Here's how the part is built. I have some questions about the finished solid (model axes, mm). Face numbers are marked on the shaded views. A direction names the side the tool comes from. Round coordinates to 2 decimals unless told otherwise and drop trailing zeros. Order: outer loops, then holes, each group sorted by start corner. A loop starts at its lowest first (then second) coordinate and runs counter-clockwise, first axis right, second up. Notation, with made-up numbers: (-18, 83.5) -> (-4, 83.5) arc R28 cw to (-4, 103.5) -> close; hole circle Ø5 at (-19, 85.5). An arc over 180 degrees is marked (long way). Use a Markdown table: item, result. Add a question column.
(1) Thinking about a two-plate mould opening in X: for the marked faces 4, 5, 6 and 7, which applies, pulls with the +X half, pulls with the -X half, needs draft (parallel to the pull), parting line crosses it, or undercut?
(2) I want a section at A-A, the plane z = 2.7. Please give me the cut outline in (x, y) (3 decimals).
(3) I want a section at B-B, the plane x = 2.75. Please give me the cut outline in (y, z).
(4) If I drill on probe 1 along Y at (x, z) = (5, 4.35) (3 decimals); probe 2 along X at (y, z) = (7.25, 2.9); probe 3 along X at (y, z) = (12.25, 3.3), over which ranges is the centre line in solid material (lowest first)?
(5) I want a section at C-C, the plane y = 11.25. Please give me the cut outline in (x, z), then the cut area to 3 significant figures.
(6) On a 3-axis mill with a long thin cutter (end or side, diameter ignored), from which of +Z, -Z, +X, -X, +Y, -Y can I reach the whole of each face in a straight line? I mean the marked faces 1, 2 and 3. Say none if no direction works.
(7) I want a section at D-D, the plane x = 5. Please give me the cut outline in (y, z) (3 decimals), then the cut area to 3 significant figures.
(8) I'm going to push flat-ended pins straight in: P1, Ø0.9, axis at y = 13.5, z = 4, coming from the -X side; P2, Ø1, axis at y = 4, z = 3, coming from the -X side; P3, Ø1.2, axis at y = 13.5, z = 2.5, coming from the +X side; P4, Ø5, axis at x = 8.5, y = 11.5, coming from the -Z side. Where does each tip first touch, or does it pass through?
from build123d import *

# Parameters (mm, degrees)
SKETCH1_R           = 3.5
BOSS_EXTRUDE1_DEPTH = 6
SKETCH2_W           = 3
SKETCH2_H           = 6
CUT_EXTRUDE1_DEPTH  = 23.414057106
FILLET1_R           = 2
FILLET2_R           = 1


with BuildPart() as part:
    # Sketch1 → Boss-Extrude1 (new body)
    with BuildSketch(Plane.XY):
        with BuildLine():
            Line((0, 3), (0, 0))
            Line((0, 0), (10, 0))
            Line((10, 0), (10, 3))
            ThreePointArc((10, 3), (5, 17.244997998), (0, 3))
        make_face()
        with Locations((5, 9.244997998)):
            Circle(SKETCH1_R, mode=Mode.SUBTRACT)
    extrude(amount=BOSS_EXTRUDE1_DEPTH)

    # Sketch2 → Cut-Extrude1 (cut, through all)
    with BuildSketch(Plane.XY.offset(6)):
        with Locations((5, 15)):
            Rectangle(SKETCH2_W, SKETCH2_H)
    extrude(amount=-CUT_EXTRUDE1_DEPTH, mode=Mode.SUBTRACT)

    # Fillet1
    fillet1_edges = [part.edges().sort_by_distance(p)[0] for p in [
        (3.5, 17.103114821, 3),
        (6.5, 17.103114821, 3),
    ]]
    fillet(fillet1_edges, radius=FILLET1_R)

    # Fillet2
    fillet2_edges = [part.edges().sort_by_distance(p)[0] for p in [
        (6.5, 12.407275659, 3),
        (3.5, 12.407275659, 3),
    ]]
    fillet(fillet2_edges, radius=FILLET2_R)


solid = part.part
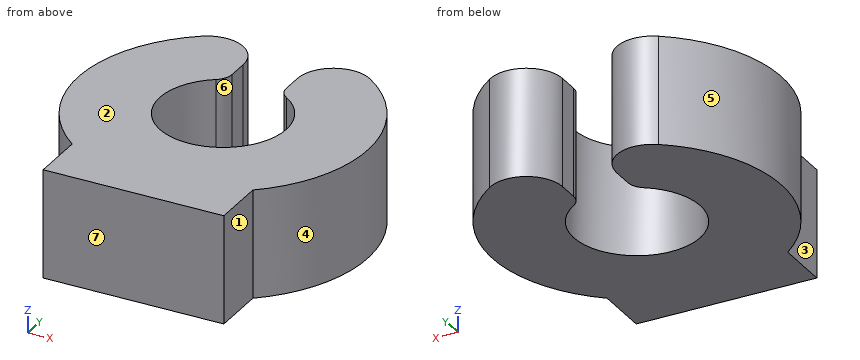
Taken from the geometry:
| question | item | result |
|---|---|---|
| 1 | face 4 | pulls with the +X half |
| 1 | face 5 | pulls with the -X half |
| 1 | face 6 | undercut |
| 1 | face 7 | needs draft |
| 2 | outline | (0, 0) -> (10, 0) -> (10, 3) arc R8 ccw to (9.667, 15.743) arc R2 ccw to (6.5, 14.118) -> (6.5, 12.987) arc R1 ccw to (6.944, 12.155) arc R3.5 cw (long way) to (3.056, 12.155) arc R1 ccw to (3.5, 12.987) -> (3.5, 14.118) arc R2 ccw to (0.333, 15.743) arc R8 ccw to (0, 3) -> close |
| 3 | outline | (0, 0) -> (6.56, 0) -> (6.56, 6) -> (0, 6) -> close; (11.93, 0) -> (15.68, 0) -> (15.68, 6) -> (11.93, 6) -> close |
| 4 | probe 1 | y = 0 to 5.745 |
| 4 | probe 2 | x = -2.75 to 2.12, 7.88 to 12.75 |
| 4 | probe 3 | x = -2.41 to 3.18, 6.82 to 12.41 |
| 5 | outline | (-2.74, 0) -> (2.13, 0) -> (2.13, 6) -> (-2.74, 6) -> close; (7.87, 0) -> (12.74, 0) -> (12.74, 6) -> (7.87, 6) -> close |
| 5 | area | 58.5 mm2 |
| 6 | face 1 | +Z, -Z, +X, -Y |
| 6 | face 2 | +Z, +X, -X, +Y, -Y |
| 6 | face 3 | +Z, -Z, -X, -Y |
| 7 | outline | (0, 0) -> (5.745, 0) -> (5.745, 6) -> (0, 6) -> close |
| 7 | area | 34.5 mm2 |
| 8 | P1 | stops at x = -2.04 |
| 8 | P2 | stops at x = -1.44 |
| 8 | P3 | stops at x = 12.12 |
| 8 | P4 | stops at z = 0 |
